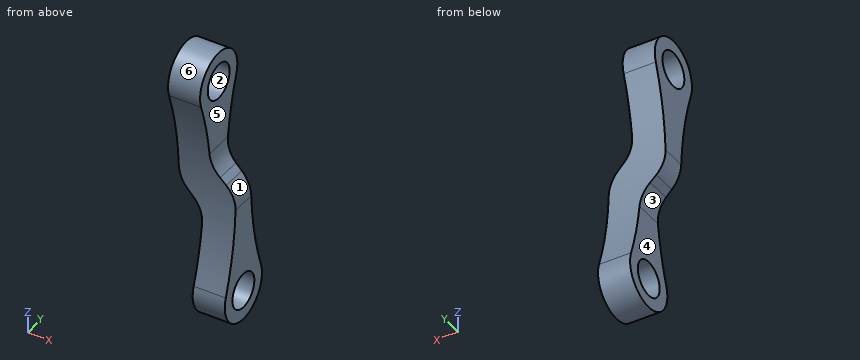
from build123d import *

# Parameters (mm, degrees)
SKETCH1_R               = 3.57
BOSS_EXTRUDE1_DEPTH     = 11.5
CUT_EXTRUDE2_DEPTH      = 51.493157952
CUT_EXTRUDE2_DEPTH_BACK = 51.493157952
FILLET1_R               = 6.5


with BuildPart() as part:
    # Sketch1 → Boss-Extrude1 (new body)
    with BuildSketch(Plane(origin=(0, 0, 0), x_dir=(0, 0, -1), z_dir=(1, 0, 0))):
        with BuildLine():
            ThreePointArc((-1.973878431, -5.740096161), (6.07, 0), (-1.973878431, 5.740096161))
            ThreePointArc((-1.973878431, 5.740096161), (-21.36, 2.5), (-40.746121569, 5.740096161))
            ThreePointArc((-40.746121569, 5.740096161), (-48.79, 0), (-40.746121569, -5.740096161))
            ThreePointArc((-40.746121569, -5.740096161), (-21.36, -2.5), (-1.973878431, -5.740096161))
        make_face()
        Circle(SKETCH1_R, mode=Mode.SUBTRACT)
        with Locations((-42.72, 0)):
            Circle(SKETCH1_R, mode=Mode.SUBTRACT)
    extrude(amount=BOSS_EXTRUDE1_DEPTH)

    # Sketch2 → Cut-Extrude2 (cut, two sides: drawn at the far end of the back side and taken through both)
    with BuildSketch(Plane(origin=(0, 0, 0), x_dir=(1, 0, 0), z_dir=(0, 1, 0)).offset(-CUT_EXTRUDE2_DEPTH_BACK)):
        Polygon((11.5, -48.79), (6.5, -48.79), (6.5, -26.36), (11.5, -21.36), align=None)
        Polygon((5, -16.30090598), (5, 6.07), (0, 6.07), (0, -21.30090598), align=None)
    extrude(amount=CUT_EXTRUDE2_DEPTH + CUT_EXTRUDE2_DEPTH_BACK, mode=Mode.SUBTRACT)

    # Fillet1
    fillet1_edges = [part.edges().sort_by_distance(p)[0] for p in [
        (0, 0, 21.30090598),
        (5, 0, 16.30090598),
        (6.5, 0, 26.36),
        (11.5, 0, 21.36),
    ]]
    fillet(fillet1_edges, radius=FILLET1_R)


solid = part.part
Could you check a few things on this model? Use its own coordinates, in mm. Face numbers are marked on the shaded views. A direction names the side the tool comes from. Coordinates: 2 decimals unless noted, no trailing zeros. Order: outer loops, then holes, each group sorted by start corner. A loop starts at its lowest first (then second) coordinate and runs counter-clockwise, first axis right, second up. Notation, with made-up numbers: (33.5, -40) -> (92.5, -40) arc R28 ccw to (92.5, -22) -> close; hole circle Ø4 at (5.25, 48). An arc over 180 degrees is marked (long way). One line per item, written item: value. Start each with the question number.
1) If I drill on L1, parallel to Y at x = 8, z = 0; L2, parallel to X at y = 0.25, z = 11; L3, parallel to Z at x = 9.75, y = 0, over which ranges is the centre line in solid material (lowest first)? Write a range as [from, to].
2) Imagine slicing it at D-D on y = 4.25. List the corners of the cut face in (x, z) for me, plus the area to 3 significant figures.
3) Which directions (+Z, -Z, +X, -X, +Y, -Y) give clear straight access to the entire face, cutting with the end or side of a thin tool? Please do the marked faces 4, 5 and 6.
4) I'm going to push flat-ended pins straight in: pin 1 (6 mm diameter, centred on x = 1.5, z = 30.5, fed in from -Y); pin 2 (2 mm diameter, centred on x = 1.5, y = -1.5, fed in from -Z); pin 3 (6 mm diameter, centred on x = 9, z = 16, fed in from -Y). Where does each tip first touch, or does it pass through?
5) Imagine slicing it at A-A on z = 42.72. List the corners of the cut face in (x, y) for me.
6) Imagine slicing it at C-C on x = 6. List the corners of the cut face in (y, z) for me, plus the area to 3 significant figures.
7) Imagine slicing it at B-B on y = 0. List the corners of the cut face in (x, z) for me, plus the area to 3 significant figures.
8) We'd pull the mould along Z, two halves only. Please class the marked faces 1, 2 and 3: +Z half, -Z half, draft (parallel to the pull), parting line (faces both ways), or undercut.
Answer list:
1. L1: y = [-6.07, -3.57], [3.57, 6.07]
1. L2: x = [5, 11.5]
1. L3: z = [-6.07, -3.57], [3.57, 23.1]
2. outline: (0, 35.7) -> (6.5, 35.7) -> (6.5, 47.05) -> (0, 47.05) -> close; (5, -4.33) -> (11.5, -4.33) -> (11.5, 7.02) -> (5, 7.02) -> close
2. area: 148 mm2
3. face 4: -Z, -X, +Y, -Y
3. face 5: +Z, +X, +Y, -Y
3. face 6: +X, -X
4. pin 1: stops at y = -3.75
4. pin 2: stops at z = 18.8
4. pin 3: stops at y = -3.09
5. outline: (0, -6.07) -> (6.5, -6.07) -> (6.5, -3.57) -> (0, -3.57) -> close; (0, 3.57) -> (6.5, 3.57) -> (6.5, 6.07) -> (0, 6.07) -> close
6. outline: (-5.74, 1.97) arc R6.07 ccw (long way) to (5.74, 1.97) arc R59.62 cw to (5.74, 40.75) arc R6.07 ccw (long way) to (-5.74, 40.75) arc R59.62 cw to start; hole circle Ø7.14 at (0, 0); hole circle Ø7.14 at (0, 42.72)
6. area: 359 mm2
7. outline: (0, 23.99) arc R6.5 ccw to (1.9, 19.4) -> (3.1, 18.2) arc R6.5 cw to (5, 13.61) -> (5, 3.57) -> (11.5, 3.57) -> (11.5, 18.67) arc R6.5 ccw to (9.6, 23.26) -> (8.4, 24.46) arc R6.5 cw to (6.5, 29.05) -> (6.5, 39.15) -> (0, 39.15) -> close; (0, 46.29) -> (6.5, 46.29) -> (6.5, 48.79) -> (0, 48.79) -> close; (5, -6.07) -> (11.5, -6.07) -> (11.5, -3.57) -> (5, -3.57) -> close
7. area: 289 mm2
8. face 1: +Z half
8. face 2: undercut
8. face 3: -Z half
